from build123d import *

# Parameters (mm, degrees)
F0_W     = 25
F0_H     = 45
F0_R     = 2
F1_DEPTH = 2


with BuildPart() as f1:
    # F0 (on Top) → F1 (new body)
    with BuildSketch(Plane.XY):
        Rectangle(F0_W, F0_H)
        with Locations((-7.5, -17.5)):
            Circle(F0_R, mode=Mode.SUBTRACT)
        with Locations((7.5, -17.5)):
            Circle(F0_R, mode=Mode.SUBTRACT)
        with Locations((-7.5, 17.5)):
            Circle(F0_R, mode=Mode.SUBTRACT)
        with BuildLine():
            ThreePointArc((-3.478162, 2.211919), (0.041681, 14.202904), (3.407455, 2.167764))
            Line((3.407455, 2.167764), (3.407455, -9.497431))
            ThreePointArc((3.407455, -9.497431), (0.207613, -13.790799), (-3.478162, -9.906592))
            Line((-3.478162, -9.906592), (-3.478162, 2.211919))
        make_face(mode=Mode.SUBTRACT)
        with Locations((7.5, 17.5)):
            Circle(F0_R, mode=Mode.SUBTRACT)
    extrude(amount=F1_DEPTH)


solid = f1.part
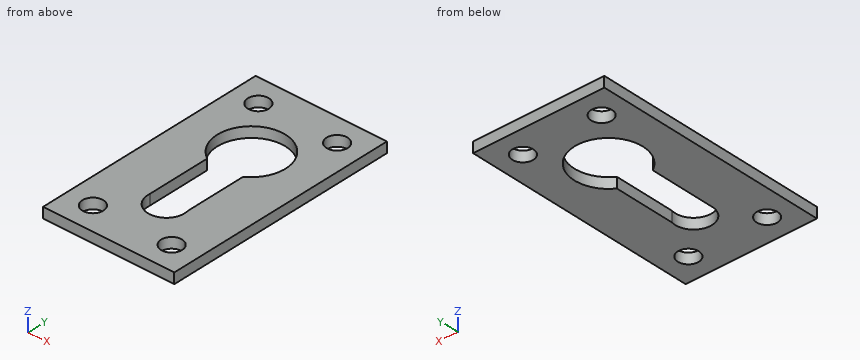
The listing builds one solid part. Answer for the finished solid, in the listing's coordinates (mm). Round coordinates to 2 decimals unless told otherwise and drop trailing zeros. Write each loop counter-clockwise with the first axis right and the second up, starting at its lowest first coordinate (ties: lowest second). Pieces come first, ordered by that corner, then holes. Notation, with made-up numbers: (18.5, 82) - (65.5, 82) arc R36 ccw to (65.5, 117) - close; hole circle Ø11 at (10.5, -23.75). An arc over 180 degrees is marked (long way). Use one line per item in the form item = value. Start each with the question number.
Item 1: A cutting plane is placed at D-D (x = 0). Write down the section's boundary in (y, z), plus the area to 3 significant figures.
Item 2: A cutting plane is placed at A-A (y = 1). Write down the section's boundary in (x, z), plus the area to 3 significant figures.
Item 3: Flat-ended cylindrical pins translate along their axes: pin 1 Ø2.5 at (x, y) = (-7.5, 17.5) entering from +Z; pin 2 Ø2 at (x, y) = (-3, -2) entering from +Z. Find the tip coordinate at first contact, or state that the pin passes through.
Item 4: A cutting plane is placed at B-B (x = 7.5). Write down the section's boundary in (y, z).
Item 5: A cutting plane is placed at C-C (y = -17.5). Write down the section's boundary in (x, z), plus the area to 3 significant figures.
Item 6: Find the intervals of material crossed by line 1 (Y direction, x = -7.5, z = 0.95); line 2 (X direction, y = -2, z = 0.85); line 3 (X direction, y = 18, z = 1.45), in increasing order. Write a range as [from, to].
The answers:
q1.outline = (-22.5, 0) - (-13.8, 0) - (-13.8, 2) - (-22.5, 2) - close; (14.2, 0) - (22.5, 0) - (22.5, 2) - (14.2, 2) - close
q1.area = 34.0 mm^2
q2.outline = (-12.5, 0) - (-3.48, 0) - (-3.48, 2) - (-12.5, 2) - close; (3.41, 0) - (12.5, 0) - (12.5, 2) - (3.41, 2) - close
q2.area = 36.2 mm^2
q3.pin_1 = through
q3.pin_2 = 2
q4.outline = (-22.5, 0) - (-19.5, 0) - (-19.5, 2) - (-22.5, 2) - close; (-15.5, 0) - (15.5, 0) - (15.5, 2) - (-15.5, 2) - close; (19.5, 0) - (22.5, 0) - (22.5, 2) - (19.5, 2) - close
q5.outline = (-12.5, 0) - (-9.5, 0) - (-9.5, 2) - (-12.5, 2) - close; (-5.5, 0) - (5.5, 0) - (5.5, 2) - (-5.5, 2) - close; (9.5, 0) - (12.5, 0) - (12.5, 2) - (9.5, 2) - close
q5.area = 34.0 mm^2
q6.line_1 = [-22.5, -19.5], [-15.5, 15.5], [19.5, 22.5]
q6.line_2 = [-12.5, -3.48], [3.41, 12.5]
q6.line_3 = [-12.5, -9.44], [-5.56, 5.56], [9.44, 12.5]
